For this review, take the finished solid that the model builds, in its own axes (mm). A direction names the side the tool comes from. Give positions to 0.01 mm unless a question says otherwise; leave off trailing zeros. Write each loop counter-clockwise with the first axis right and the second up, starting at its lowest first coordinate (ties: lowest second). Pieces come first, ordered by that corner, then holes.
Q1. We need section D-D (y = -16.5). Write out the cut boundary in (x, z), then the cut area to 3 significant figures.
Q2. Machinability: for faces 1 (the flat face through (-1, 32.846, 13)), 2 (the flat face through (-13, 8, 25.4)), which of the approach directions +Z, -Z, +X, -X, +Y, -Y give a long, thin tool a straight path to every point of the face, cutting with its end or side? Answer none if there is none.
Q3. We need section C-C (z = 39.5). Write out the cut boundary in (x, y), then the cut area to 3 significant figures.
Q4. We need section B-B (x = 1.5). Write out the cut boundary in (y, z).
Q5. We need section A-A (y = 0). Write out the cut boundary in (x, z).
Q6. For line 1 (Z direction, x = 2.5, y = -28.5); line 2 (X direction, y = -11, z = 47); line 3 (Z direction, x = 10, y = 4), list the stretches that pass through material, from the lowest coordinate up.
Q7. Insertion check: P1, Ø1.5, axis at x = 24, y = 16.5, coming from the +Z side; P2, Ø10, axis at y = -1.5, z = 34, coming from the -X side. Each pin has a flat end and moves straight along its axis. Give the tip position at first contact, or say it passes through.
```python
from build123d import *

# Parameters (mm, degrees)
F0_W     = 110.738724
F0_H     = 65.69177
F1_DEPTH = 25.4
F2_R     = 14.059136
F3_DEPTH = 50.8
F5_DEPTH = 50.8
F7_DEPTH = 25.4


with BuildPart() as f1:
    # F0 (on Top) → F1 (new body)
    with BuildSketch(Plane.XY):
        Rectangle(F0_W, F0_H)
    extrude(amount=F1_DEPTH)

    # F2 (on face) → F3 (join)
    with BuildSketch(Plane.XY.offset(25.4)):
        Circle(F2_R)
    extrude(amount=F3_DEPTH)

    # F4 (on Front) → F5 (cut, symmetric)
    with BuildSketch(Plane.XZ):
        Polygon((27.752033, 54.067187), (-22.952005, 54.067187), (27.752033, 29.959714), align=None)
    extrude(amount=F5_DEPTH, both=True, mode=Mode.SUBTRACT)

    # F6 (on Front) → F7 (cut, symmetric)
    with BuildSketch(Plane.XZ):
        Polygon((-32.981899, 81.521302), (-32.981899, 52.895501), (34.759905, 52.895501), (27.647903, 81.521302), align=None)
    extrude(amount=F7_DEPTH, both=True, mode=Mode.SUBTRACT)


solid = f1.part
```
Computed:
1. outline: (-55.37, 0) - (55.37, 0) - (55.37, 25.4) - (-55.37, 25.4) - close
1. area: 2,810 mm2
2. face 1: +Z, -Z, +X, -X, +Y
2. face 2: +Z
3. outline: (7.69, -11.77) - (7.69, 11.77) arc R14.06 ccw (long way) to start
3. area: 515 mm2
4. outline: (-32.85, 0) - (32.85, 0) - (32.85, 25.4) - (13.98, 25.4) - (13.98, 42.44) - (-13.98, 42.44) - (-13.98, 25.4) - (-32.85, 25.4) - close
5. outline: (-55.37, 0) - (55.37, 0) - (55.37, 25.4) - (14.06, 25.4) - (14.06, 36.47) - (-14.06, 49.84) - (-14.06, 25.4) - (-55.37, 25.4) - close
6. line 1: z = 0 to 25.4
6. line 2: x = -8.76 to -8.09
6. line 3: z = 0 to 38.4
7. P1: stops at z = 25.4
7. P2: stops at x = -14.06
